The model under review builds one solid part; all positions refer to its coordinate system, in mm. Face numbers are marked on the shaded views. A direction names the side the tool comes from. Coordinates: 2 decimals unless noted, no trailing zeros. Order: outer loops, then holes, each group sorted by start corner. A loop starts at its lowest first (then second) coordinate and runs counter-clockwise, first axis right, second up.
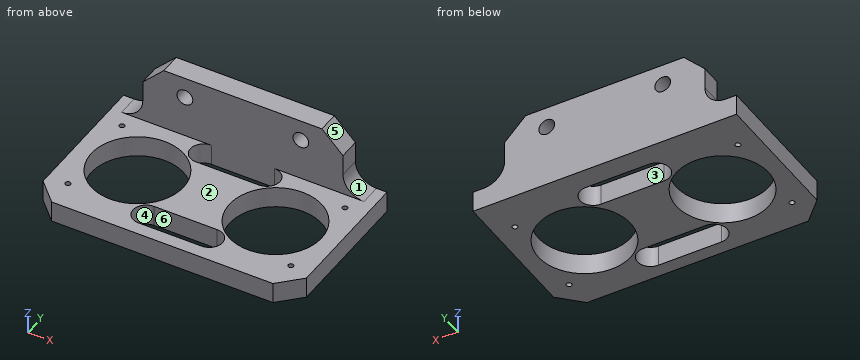
```python
from build123d import *

# Parameters (mm, degrees)
SKETCH_R             = 1.5
PAD_DEPTH            = 4
SKETCH001_R          = 0.5
SKETCH001_R_2        = 8.75
PAD001_DEPTH         = 4
FILLET_R             = 4
CHAMFER_SIZE         = 4
BODY_PLACEMENT_ANGLE = 90


with BuildPart() as part:
    # Sketch → Pad (new body)
    with BuildSketch(Plane.XY):
        Polygon((-15, 4), (15, 4), (19, 0), (19, -8), (-19, -8), (-19, 0), align=None)
        with Locations((-11, 0)):
            Circle(SKETCH_R, mode=Mode.SUBTRACT)
        with Locations((11, 0)):
            Circle(SKETCH_R, mode=Mode.SUBTRACT)
    extrude(amount=PAD_DEPTH)

    # Sketch001 (on Face2 of Pad) → Pad001 (join)
    with BuildSketch(Plane.XZ.offset(8)):
        Polygon((-25, 30), (25, 30), (25, 0), (0, 0), (-25, 0), align=None)
        with Locations((-21.15, 24.5)):
            Circle(SKETCH001_R, mode=Mode.SUBTRACT)
        with Locations((-21.15, 7)):
            Circle(SKETCH001_R, mode=Mode.SUBTRACT)
        with Locations((21.15, 7)):
            Circle(SKETCH001_R, mode=Mode.SUBTRACT)
        with Locations((21.15, 24.5)):
            Circle(SKETCH001_R, mode=Mode.SUBTRACT)
        with Locations((-13.1, 15.75)):
            Circle(SKETCH001_R_2, mode=Mode.SUBTRACT)
        with Locations((13.1, 15.75)):
            Circle(SKETCH001_R_2, mode=Mode.SUBTRACT)
        with BuildLine():
            Line((-6, 4), (0, 4))
            Line((6, 4), (0, 4))
            ThreePointArc((6, 4), (8.5, 6.5), (6, 9))
            Line((-6, 9), (6, 9))
            ThreePointArc((-6, 9), (-8.5, 6.5), (-6, 4))
        make_face(mode=Mode.SUBTRACT)
        with BuildLine():
            Line((-6, 27.5), (0, 27.5))
            Line((0, 27.5), (6, 27.5))
            ThreePointArc((6, 22.5), (8.5, 25), (6, 27.5))
            Line((-6, 22.5), (6, 22.5))
            ThreePointArc((-6, 27.5), (-8.5, 25), (-6, 22.5))
        make_face(mode=Mode.SUBTRACT)
    extrude(amount=PAD001_DEPTH)

    # Fillet
    fillet_edges = [part.edges().sort_by_distance(p)[0] for p in [
        (19, -8, 2),
        (-19, -8, 2),
    ]]
    fillet(fillet_edges, radius=FILLET_R)

    # Chamfer
    chamfer_edges = [part.edges().sort_by_distance(p)[0] for p in [
        (-25, -10, 30),
        (25, -10, 30),
    ]]
    chamfer(chamfer_edges, length=CHAMFER_SIZE)


with BuildPart() as part_1:
    # Body placement: moved
    add(part.part.rotate(Axis((0, 0, 0), (1, 0, 0)), BODY_PLACEMENT_ANGLE))


solid = part_1.part
```
(1) We need section C-C, the plane z = -10. Count the separate pieces of the cut face and the enclosed holes in it, and give its area (3 significant figures).
A:
separate pieces: 1
enclosed holes: 8
area: 841 mm2
(2) Draft analysis for pull direction X (two halves, no side actions). For the marked faces 1, 2, 3 and 4, state which applies: released by +X, released by -X, zero draft, split by the parting line, or undercut.
A:
face 1: released by +X
face 2: zero draft
face 3: undercut
face 4: undercut
(3) Machinability: for the marked faces 5 and 6, which of the approach directions +Z, -Z, +X, -X, +Y, -Y give a long, thin tool a straight path to every point of the face, cutting with its end or side? Answer none if there is none.
A:
face 5: +Z, +X, +Y, -Y
face 6: +Z, -Z
(4) We need section B-B, the plane x = -2. Write out the cut boundary in (y, z).
A:
outline: (-30, -12) - (-27.5, -12) - (-27.5, -8) - (-30, -8) - close; (-22.5, -12) - (-9, -12) - (-9, -8) - (-22.5, -8) - close; (-4, -12) - (0, -12) - (0, 4) - (-4, 4) - close
(5) We need section A-A, the plane y = -15.75. Write out the cut boundary in (x, z), and give its area (3 significant figures).
A:
outline: (-25, -12) - (-21.85, -12) - (-21.85, -8) - (-25, -8) - close; (-4.35, -12) - (4.35, -12) - (4.35, -8) - (-4.35, -8) - close; (21.85, -12) - (25, -12) - (25, -8) - (21.85, -8) - close
area: 60.0 mm2
(6) We need section D-D, the plane x = 13.1. Write out the cut boundary in (y, z).
A:
outline: (-30, -12) - (-24.5, -12) - (-24.5, -8) - (-30, -8) - close; (-7, -12) - (0, -12) - (0, 4) - (-4, 4) - (-4, -8) - (-7, -8) - close
(7) Wall thickness on probe 1 along X at (y, z) = (-15.75, -9.75); probe 2 along Y at (x, z) = (-2.5, -11); probe 3 along Y at (x, z) = (-21.15, -10.8): over which ranges is each line inside the solid? List them lowest first.
A:
probe 1: x = -25 to -21.85, -4.35 to 4.35, 21.85 to 25
probe 2: y = -30 to -27.5, -22.5 to -9, -4 to 0
probe 3: y = -29.85 to -25, -24 to -19.18, -12.32 to -7.5, -6.5 to 0
(8) For pin 1 Ø6 at (y, z) = (-6, -1.5) entering from -X; pin 2 Ø1.8 at (x, z) = (-11, 0) entering from -Y; pin 3 Ø8 at (x, y) = (-6.5, -22.5) entering from +Z; pin 4 Ø3 at (x, z) = (13, 1) entering from -Y, all flat-tipped, find the tip position at first contact; note any pin that passes through.
A:
pin 1: stops at x = -19
pin 2: passes through
pin 3: stops at z = -8
pin 4: stops at y = -4
